Answer from the drawing. Dimensions are ordinates in mm from the lowest x, y and z of the part. A direction names the side the tool comes from. Round coordinates to 2 decimals unless told otherwise and drop trailing zeros. Order: outer loops, then holes, each group sorted by start corner. A loop starts at its lowest first (then second) coordinate and runs counter-clockwise, first axis right, second up. Notation, with made-up numbers: (8, -24.75) -> (55, -24.75) arc R19 cw to (55, -19.75) -> close; hole circle Ø10 at (-34, 85). An arc over 180 degrees is marked (long way). Use a Markdown table: item, result. Add a question column.
1. Given pin 1 (9.5 mm diameter, centred on x = 10.5, z = 4.5, fed in from -Y); pin 2 (2 mm diameter, centred on x = 16, y = 17.5, fed in from -Z); pin 3 (6 mm diameter, centred on x = 10, y = 5.5, fed in from -Z), each flat-ended and moving along its own axis, determine where each tip first touches the part or whether it passes through.
2. The mould has two halves that part along X. Classify the marked faces 4, 5 and 6: +X half, -X half, draft (parallel to the pull), parting line (faces both ways), or undercut.
3. Section C-C, the plane z = 29 is taken. Give the vertices of the cut face in (x, y).
4. Consider L1, parallel to X at y = 1.15, z = 26; L2, parallel to X at y = 24.65, z = 4; L3, parallel to X at y = 22.75, z = 1.5. Determine where each line is inside the solid, lowest interval first. Write a range as [from, to].
5. For the marked faces 1, 2 and 3, determine the directions among +Z, -Z, +X, -X, +Y, -Y from which every point of the face is accessible in a straight line to the end or side of a thin tool.
6. Section B-B, the plane x = 18 is taken. Give the vertices of the cut face in (y, z), then the cut area to 3 significant figures.
7. Section D-D, the plane x = 10.5 is taken. Give the vertices of the cut face in (y, z), then the cut area to 3 significant figures.
8. Section A-A, the plane z = 5 is taken. Give the vertices of the cut face in (x, y), then the cut area to 3 significant figures.
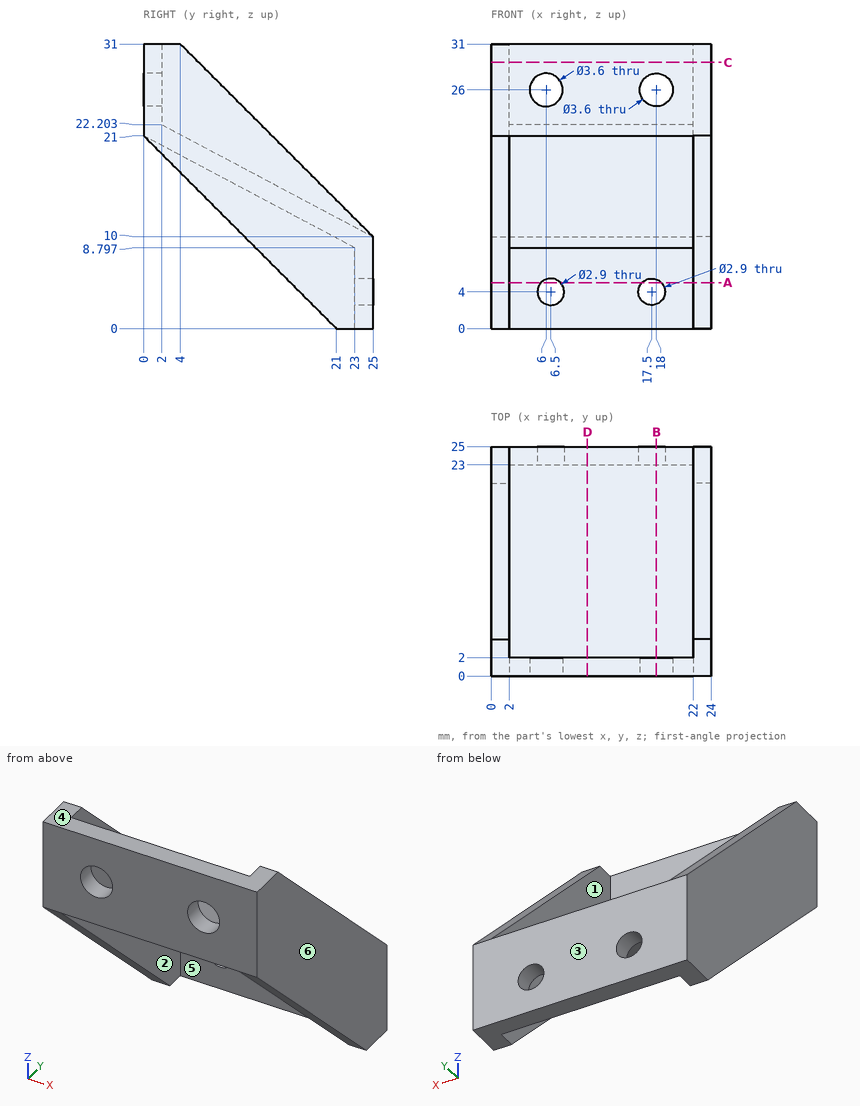
Verdict:
| question | item | result |
|---|---|---|
| 1 | pin 1 | stops at y = 22.15 |
| 1 | pin 2 | stops at z = 11.18 |
| 1 | pin 3 | stops at z = 16.49 |
| 2 | face 4 | draft |
| 2 | face 5 | undercut |
| 2 | face 6 | +X half |
| 3 | outline | (0, 0) -> (24, 0) -> (24, 6) -> (22, 6) -> (22, 2) -> (2, 2) -> (2, 6) -> (0, 6) -> close |
| 4 | L1 | x = [0, 4.2], [7.8, 16.2], [19.8, 24] |
| 4 | L2 | x = [0, 5.05], [7.95, 16.05], [18.95, 24] |
| 4 | L3 | x = [0, 2], [22, 24] |
| 5 | face 1 | +Z, +Y |
| 5 | face 2 | -Z, -Y |
| 5 | face 3 | +Z, -Z, +X, -X, +Y |
| 6 | outline | (0, 21) -> (23, 8.8) -> (23, 5.36) -> (25, 5.36) -> (25, 10) -> (2, 22.2) -> (2, 24.2) -> (0, 24.2) -> close; (0, 27.8) -> (2, 27.8) -> (2, 31) -> (0, 31) -> close; (23, 0) -> (25, 0) -> (25, 2.64) -> (23, 2.64) -> close |
| 6 | area | 77.0 mm2 |
| 7 | outline | (0, 21) -> (23, 8.8) -> (23, 0) -> (25, 0) -> (25, 10) -> (2, 22.2) -> (2, 31) -> (0, 31) -> close |
| 7 | area | 89.7 mm2 |
| 8 | outline | (0, 16) -> (2, 16) -> (2, 23) -> (5.45, 23) -> (5.45, 25) -> (0, 25) -> close; (7.55, 23) -> (16.45, 23) -> (16.45, 25) -> (7.55, 25) -> close; (18.55, 23) -> (22, 23) -> (22, 16) -> (24, 16) -> (24, 25) -> (18.55, 25) -> close |
| 8 | area | 67.6 mm2 |
